Autodesk Fusion 360 part; units mm, degrees
sketch "Sketch1" plane through (0, 0, 0) normal (0, 0, 1) x (1, 0, 0)
  line L0 (0, 0) -> (98, 0)
  line L1 (98, 0) -> (98, 150)
  line L2 (98, 150) -> (0, 150)
  line L3 (0, 150) -> (0, 0)
  dimension "d1" = 98
  dimension "d2" = 150
extrude "Extrude1" add sketch "Sketch1" along normal blind 45
sketch "Sketch2" plane through (0, 0, 45) normal (0, 0, 1) x (-1, 0, 0)
  line L0 (0, -150) -> (0, 0)
  line L1 (0, 0) -> (-98, 0)
  line L2 (-98, 0) -> (-98, -150)
  line L3 (-98, -150) -> (0, -150)
  line L4 (0, 0) -> (-2.5, 0)
  line L5 (-2.5, 0) -> (-2.5, -2.5)
  line L6 (-2.5, -2.5) -> (-95.5, -2.5)
  line L7 (-95.5, -2.5) -> (-95.5, -147.5)
  line L8 (-95.5, -147.5) -> (-2.5, -147.5)
  line L9 (-2.5, -147.5) -> (-2.5, -2.5)
  dimension "d5" = 2.5
  dimension "d6" = 2.5
  dimension "d7" = 93
  dimension "d8" = 145
extrude "Extrude2" cut sketch "Sketch2" against normal blind 42.5 contours L6 L7 L8 L9
extrude "Extrude3" cut 1 faces at (2.5, 99.1667, 16.6667) along direction (-1, 0, 0) blind 2.5
sketch "Sketch3" plane through (95.5, 0, 0) normal (-1, 0, 0) x (0, -1, 0)
  line L0 (-2.5, 45) -> (-147.5, 45)
  line L1 (-147.5, 45) -> (-147.5, 2.5)
  line L2 (-147.5, 2.5) -> (-2.5, 2.5)
  line L3 (-2.5, 2.5) -> (-2.5, 45)
sketch "Sketch4" plane through (0, 147.5, 0) normal (0, -1, 0) x (1, 0, 0)
  line L0 (95.5, 45) -> (0, 45)
  line L1 (0, 45) -> (0, 2.5)
  line L2 (0, 2.5) -> (95.5, 2.5)
  line L3 (95.5, 2.5) -> (95.5, 45)
  line L4 (0, 0) -> (97.9689, 19.9489)
extrude "Extrude4" add sketch "Sketch4" along normal blind 145 contours L2 L3 L4
sketch "Sketch7" plane through (0, 0, 45) normal (0, 0, 1) x (-1, 0, 0)
  line L0 (0, -147.5) -> (-95.5, -147.5)
  line L1 (-95.5, -147.5) -> (-95.5, -2.5)
  line L2 (-95.5, -2.5) -> (0, -2.5)
  line L3 (0, -2.5) -> (0, 0)
  line L4 (0, 0) -> (-98, 0)
  line L5 (-98, 0) -> (-98, -150)
  line L6 (-98, -150) -> (0, -150)
  line L7 (0, -150) -> (0, -147.5)
  line L8 (-98, 0) -> (0, 0)
  line L9 (0, 0) -> (0, -150)
  line L10 (0, -150) -> (-98, -150)
  line L11 (-98, -150) -> (-98, 0)
  dimension "d19" = 98
  dimension "d20" = 150
extrude "Extrude5" add sketch "Sketch7" along normal blind 2.5
fillet "Fillet1" [suppressed]
fillet "Fillet2" [suppressed]
sketch "Sketch5" plane through (95.5, 0, 0) normal (-1, 0, 0) x (0, -1, 0)
sketch "Sketch6" plane through (95.5, 0, 0) normal (-1, 0, 0) x (0, -1, 0)
Input: part model. Units: mm. Frame: model coordinates. A direction names the side the tool comes from. Coordinates: 2 decimals unless noted, no trailing zeros. Loops run counter-clockwise (first coordinate to the right, second up) from the corner with the lowest first, then second, coordinate; pieces in that order, holes last. Notation, with made-up numbers: M 89,41 L 107,41 A18 ccw 107,71 Z; hole C 28.5,25.5 d11. An arc over 180 degrees is marked long. One line per item, written item: value.
(1) Section C-C (y = 109.5). Output: boundary loops of the cut face in (x, z), and give its area (3 significant figures).
Filled in:
outline: M 0,0 L 98,0 L 98,47.5 L 0,47.5 L 0,45 L 95.5,45 L 95.5,19.45 L 12.28,2.5 L 0,2.5 Z
area: 1,300 mm^2
(2) Section D-D (z = 7). Output: boundary loops of the cut face in (x, y), and give its area (3 significant figures).
Filled in:
outline: M 0,0 L 98,0 L 98,150 L 0,150 L 0,147.5 L 34.38,147.5 L 34.38,2.5 L 0,2.5 Z
area: 9,720 mm^2
(3) Pin query (flat end, axial travel): pin 1 (10 mm diameter, centred on y = 53.5, z = 26, fed in from -X). Return the tip coordinate at first contact, or that it passes through.
Filled in:
pin 1: x = 95.5
(4) Reachability of faces 1 (the flat face through (48, 0, 23)), 2 (the flat face through (48, 147.5, 29)) from +Z, -Z, +X, -X, +Y, -Y: full face, straight path, thin tool, end or side. Return the list, or none.
Filled in:
face 1: +Z, -Z, +X, -X, -Y
face 2: -X
(5) Pull-direction query (Z, two-part tool) for faces 3 (the flat face through (48, 74, 45)), 4 (the flat face through (0, 98, 47)), 5 (the flat face through (50, 74, 47.5)), 6 (the flat face through (95.5, 74, 32)); classes: +Z half, -Z half, draft (parallel to the pull), parting line (faces both ways), or undercut.
Filled in:
face 3: undercut
face 4: draft
face 5: +Z half
face 6: undercut
(6) Line query: line 1 along Y through (x, z) = (43, 12.5); line 2 along Z through (x, y) = (5.5, 15.5); line 3 along X through (y, z) = (66, 38). Output: solid intervals per line, ascending. Write a range as from..to.
Filled in:
line 1: 0..2.5, 147.5..150
line 2: 0..2.5, 45..47.5
line 3: 95.5..98
(7) Section B-B (x = 7.5). Output: boundary loops of the cut face in (y, z), and give its area (4 significant figures).
Filled in:
outline: M 0,0 L 150,0 L 150,47.5 L 0,47.5 Z; hole M 2.5,2.5 L 147.5,2.5 L 147.5,45 L 2.5,45 Z
area: 962.5 mm^2
(8) Section A-A (z = 33). Output: boundary loops of the cut face in (x, y).
Filled in:
outline: M 0,0 L 98,0 L 98,150 L 0,150 L 0,147.5 L 95.5,147.5 L 95.5,2.5 L 0,2.5 Z
